The drawing under review shows one solid part. Ordinate dimensions are in mm from its lowest x, y, z. Give positions to 0.01 mm unless a question says otherwise; leave off trailing zeros. Loops run counter-clockwise (first coordinate to the right, second up) from the corner with the lowest first, then second, coordinate; pieces in that order, holes last. Notation, with made-up numbers: (-3.5, 57.5) - (23.5, 57.5) arc R12 cw to (23.5, 69.5) - close; hole circle Ø2 at (-10, 9). An arc over 180 degrees is marked (long way). Write each question's results on one line, items separated by ' | '.
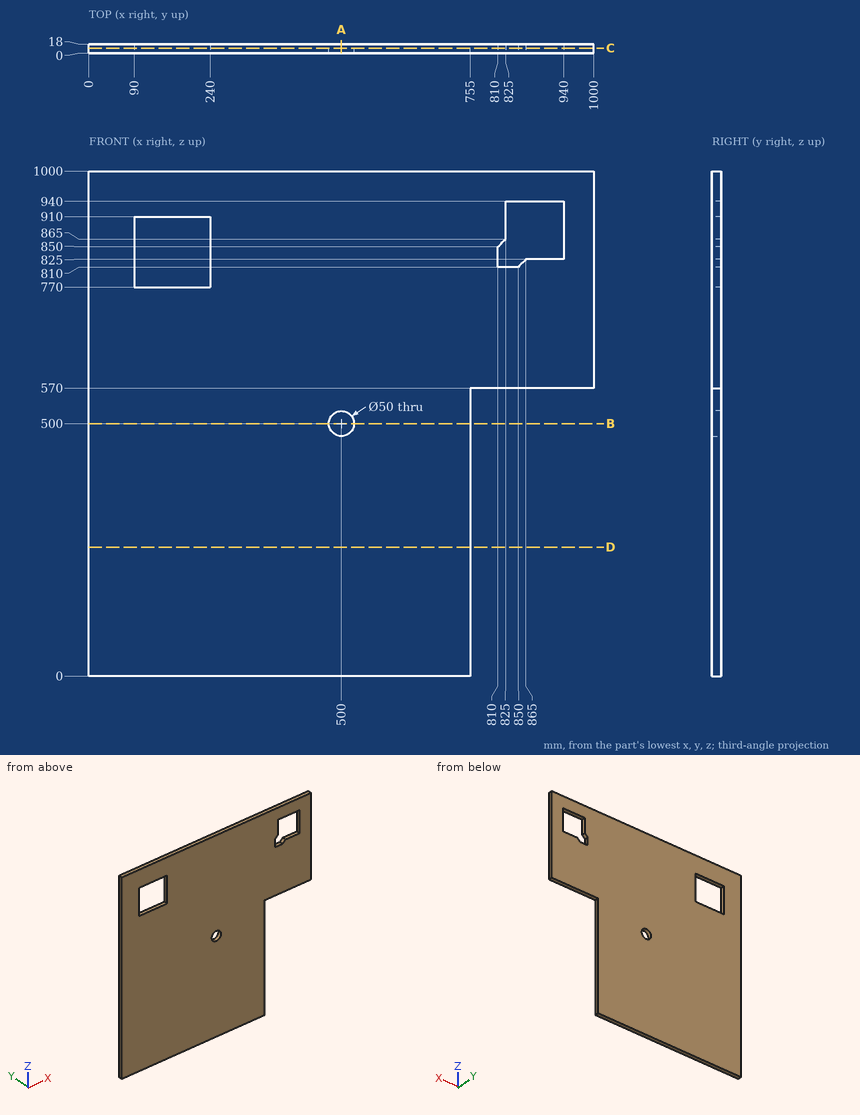
(1) Take a section at A-A on x = 500. Give the boundary of the cut face in (y, z).
Answers below:
outline: (0, 0) - (18, 0) - (18, 475) - (0, 475) - close; (0, 525) - (18, 525) - (18, 1000) - (0, 1000) - close
(2) Wall thickness on line 1 along X through (y, z) = (6.25, 500); line 2 along X through (y, z) = (17.25, 556): over which ranges is each line inside the solid? List them lowest first. Write a range as from..to.
Answers below:
line 1: 0..475, 525..755 | line 2: 0..755
(3) Insertion check: P1, Ø10, axis at y = 8.5, z = 358.5, coming from the -X side; P2, Ø8, axis at y = 12.5, z = 282.5, coming from the +X side. Each pin has a flat end and moves straight along its axis. Give the tip position at first contact, or say it passes through.
Answers below:
P1: x = 0 | P2: x = 755
(4) Take a section at B-B on z = 500. Give the boundary of the cut face in (x, y).
Answers below:
outline: (0, 0) - (475, 0) - (475, 18) - (0, 18) - close; (525, 0) - (755, 0) - (755, 18) - (525, 18) - close
(5) Take a section at C-C on y = 10. Give the boundary of the cut face in (x, z), plus the area to 3 significant figures.
Answers below:
outline: (0, 0) - (755, 0) - (755, 570) - (1000, 570) - (1000, 1000) - (0, 1000) - close; hole (90, 770) - (240, 770) - (240, 910) - (90, 910) - close; hole circle Ø50 at (500, 500); hole (810, 810) - (850, 810) - (865, 825) - (940, 825) - (940, 940) - (825, 940) - (825, 865) - (810, 850) - close | area: 823,000 mm2
(6) Take a section at D-D on z = 255. Give the boundary of the cut face in (x, y), plus the area to 3 significant figures.
Answers below:
outline: (0, 0) - (755, 0) - (755, 18) - (0, 18) - close | area: 13,600 mm2
